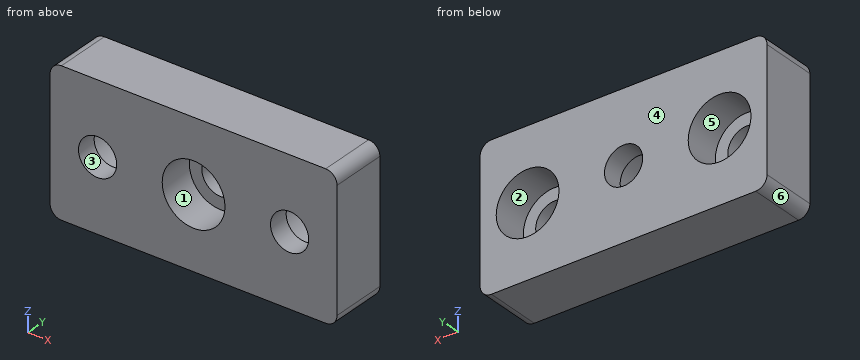
from build123d import *

# Parameters (mm, degrees)
SKETCH1_W                                        = 50.8
SKETCH1_H                                        = 25.4
BOSS_EXTRUDE1_DEPTH                              = 10
CBORE_FOR_1_4_SOCKET_HEAD_CAP_SCREW2_D           = 6.7564
CBORE_FOR_1_4_SOCKET_HEAD_CAP_SCREW2_CBORE_D     = 11.1125
CBORE_FOR_1_4_SOCKET_HEAD_CAP_SCREW2_CBORE_DEPTH = 6.35
CBORE_FOR_1_4_SOCKET_HEAD_CAP_SCREW3_D           = 6.7564
CBORE_FOR_1_4_SOCKET_HEAD_CAP_SCREW3_CBORE_D     = 11.1125
CBORE_FOR_1_4_SOCKET_HEAD_CAP_SCREW3_CBORE_DEPTH = 6.35
FILLET2_R                                        = 2


with BuildPart() as part:
    # Sketch1 → Boss-Extrude1 (new body)
    with BuildSketch(Plane(origin=(0, 0, 0), x_dir=(1, 0, 0), z_dir=(0, 1, 0))):
        with Locations((-10.671863118, -7.895247148)):
            Rectangle(SKETCH1_W, SKETCH1_H)
    extrude(amount=BOSS_EXTRUDE1_DEPTH)

    # CBORE for 1/4 Socket Head Cap Screw2 (through all)
    with Locations(Plane(origin=(0, 10, 0), x_dir=(1, 0, 0), z_dir=(0, 1, 0))):
        with Locations((-27.671863118, -7.895247148), (6.328136882, -7.895247148)):
            CounterBoreHole(CBORE_FOR_1_4_SOCKET_HEAD_CAP_SCREW2_D / 2, CBORE_FOR_1_4_SOCKET_HEAD_CAP_SCREW2_CBORE_D / 2, CBORE_FOR_1_4_SOCKET_HEAD_CAP_SCREW2_CBORE_DEPTH)

    # CBORE for 1/4 Socket Head Cap Screw3 (through all)
    with Locations(Plane(origin=(0, 0, 0), x_dir=(-1, 0, 0), z_dir=(0, -1, 0))):
        with Locations((10.671863118, -7.895247148)):
            CounterBoreHole(CBORE_FOR_1_4_SOCKET_HEAD_CAP_SCREW3_D / 2, CBORE_FOR_1_4_SOCKET_HEAD_CAP_SCREW3_CBORE_D / 2, CBORE_FOR_1_4_SOCKET_HEAD_CAP_SCREW3_CBORE_DEPTH)

    # Fillet2
    fillet2_edges = [part.edges().sort_by_distance(p)[0] for p in [
        (-36.071863118, 5, -4.804752852),
        (14.728136882, 5, -4.804752852),
        (14.728136882, 5, 20.595247148),
        (-36.071863118, 5, 20.595247148),
    ]]
    fillet(fillet2_edges, radius=FILLET2_R)


solid = part.part
Geometry check sheet. Reference: the model listing, model coordinates, mm. Face numbers are marked on the shaded views. A direction names the side the tool comes from. Round coordinates to 2 decimals unless told otherwise and drop trailing zeros. Write each loop counter-clockwise with the first axis right and the second up, starting at its lowest first coordinate (ties: lowest second). Pieces come first, ordered by that corner, then holes.
Item 1: Mould release check, pull along Z, two halves, no side actions. Record for the marked faces 4, 5 and 6: +Z half, -Z half, draft (parallel to the pull), parting line (faces both ways), or undercut.
Determined:
face 4: draft
face 5: undercut
face 6: -Z half
Item 2: Section check A-A (z = 6). Record the boundary of the cut face in (x, y), plus the area to 3 significant figures.
Determined:
outline: (-36.07, 0) - (-30.47, 0) - (-30.47, 3.65) - (-32.89, 3.65) - (-32.89, 10) - (-36.07, 10) - close; (-24.88, 0) - (-15.89, 0) - (-15.89, 6.35) - (-13.47, 6.35) - (-13.47, 10) - (-22.45, 10) - (-22.45, 3.65) - (-24.88, 3.65) - close; (-7.88, 6.35) - (-5.45, 6.35) - (-5.45, 0) - (3.53, 0) - (3.53, 3.65) - (1.11, 3.65) - (1.11, 10) - (-7.88, 10) - close; (9.12, 0) - (14.73, 0) - (14.73, 10) - (11.55, 10) - (11.55, 3.65) - (9.12, 3.65) - close
area: 248 mm2
Item 3: Section check B-B (x = 4). Record the boundary of the cut face in (y, z), plus the area to 3 significant figures.
Determined:
outline: (0, -4.8) - (10, -4.8) - (10, 2.85) - (3.65, 2.85) - (3.65, 5.45) - (0, 5.45) - close; (0, 10.34) - (3.65, 10.34) - (3.65, 12.94) - (10, 12.94) - (10, 20.6) - (0, 20.6) - close
area: 172 mm2
Item 4: Section check D-D (x = -28.5). Record the boundary of the cut face in (y, z), plus the area to 3 significant figures.
Determined:
outline: (0, -4.8) - (10, -4.8) - (10, 2.4) - (3.65, 2.4) - (3.65, 4.62) - (0, 4.62) - close; (0, 11.17) - (3.65, 11.17) - (3.65, 13.39) - (10, 13.39) - (10, 20.6) - (0, 20.6) - close
area: 160 mm2
Item 5: Section check C-C (y = 7.25). Record the boundary of the cut face in (x, z).
Determined:
outline: (-36.07, -2.8) arc R2 ccw to (-34.07, -4.8) - (12.73, -4.8) arc R2 ccw to (14.73, -2.8) - (14.73, 18.6) arc R2 ccw to (12.73, 20.6) - (-34.07, 20.6) arc R2 ccw to (-36.07, 18.6) - close; hole circle Ø11.11 at (-27.67, 7.9); hole circle Ø6.76 at (-10.67, 7.9); hole circle Ø11.11 at (6.33, 7.9)
Item 6: Material ranges on line 1 along X through (y, z) = (8.25, 8); line 2 along X through (y, z) = (6.25, 2.75); line 3 along X through (y, z) = (7.25, 4), recorded low to high.
Determined:
line 1: x = -36.07 to -33.23, -22.12 to -14.05, -7.3 to 0.77, 11.88 to 14.73
line 2: x = -36.07 to -29.77, -25.57 to -12.77, -8.57 to 4.23, 8.43 to 14.73
line 3: x = -36.07 to -31.63, -23.71 to 2.37, 10.29 to 14.73
Item 7: Access from +Z, -Z, +X, -X, +Y, -Y to the whole of each face (thin tool, end or side, straight path). Record for the marked faces 1, 2 and 3.
Determined:
face 1: -Y
face 2: +Y
face 3: +Y, -Y
Item 8: Go/stop test with flat-tipped pins: pin 1 Ø8 at (x, z) = (6.33, 7.9) entering from +Y; pin 2 Ø9 at (x, z) = (-10.67, 7.9) entering from -Y. Record where each tip stops, or that it passes through.
Determined:
pin 1: stops at y = 3.65
pin 2: stops at y = 6.35
